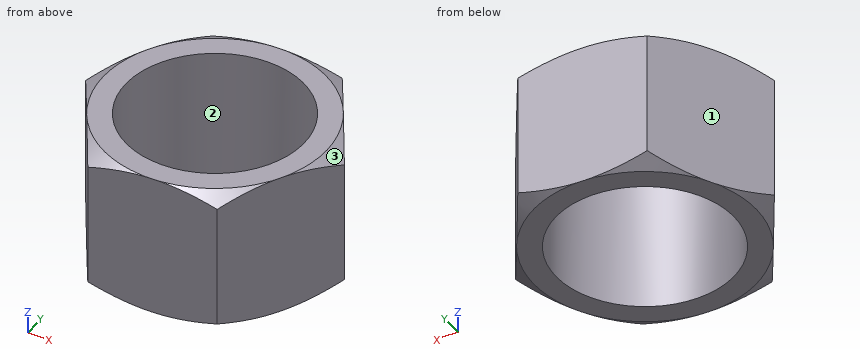
from build123d import *

# Parameters (mm, degrees)
SKETCH1_R           = 5
BOSS_EXTRUDE1_DEPTH = 8
SKETCH2_OUTSIDE_W   = 67.404
SKETCH2_OUTSIDE_H   = 65.714
SKETCH2_OUTSIDE_R   = 6.25
CUT_EXTRUDE1_DEPTH  = 13.512942035
CUT_EXTRUDE1_DRAFT  = -60
SKETCH3_OUTSIDE_W   = 67.404
SKETCH3_OUTSIDE_H   = 65.714
SKETCH3_OUTSIDE_R   = 6.251224569
CUT_EXTRUDE2_DEPTH  = 13.512942035
CUT_EXTRUDE2_DRAFT  = -60


with BuildPart() as part:
    # Sketch1 → Boss-Extrude1 (new body)
    with BuildSketch(Plane.XY):
        Polygon((3.396178054, 6.367833851), (-3.816616855, 6.125093396), (-7.212794909, -0.242740455), (-3.396178054, -6.367833851), (3.816616855, -6.125093396), (7.212794909, 0.242740455), align=None)
        Circle(SKETCH1_R, mode=Mode.SUBTRACT)
    extrude(amount=BOSS_EXTRUDE1_DEPTH)


with BuildPart() as cut_extrude1_tool:
    # Sketch2 outside → Cut-Extrude1 (with draft: the straight prism first)
    with BuildSketch(Plane.XY.offset(8)):
        Rectangle(SKETCH2_OUTSIDE_W, SKETCH2_OUTSIDE_H)
        Circle(SKETCH2_OUTSIDE_R, mode=Mode.SUBTRACT)
    extrude(amount=-CUT_EXTRUDE1_DEPTH)
    # Cut-Extrude1: the draft: its side faces are tilted about the plane it starts from
    cut_extrude1_sides = [cut_extrude1_tool.faces().sort_by_distance(p)[0] for p in [
        (0, -32.857, 1.243528983),
        (33.702, 0, 1.243528983),
        (0, 32.857, 1.243528983),
        (-33.702, 0, 1.243528983),
        (-6.25, 0, 1.243528983),
    ]]
    draft(cut_extrude1_sides, Plane.XY.offset(8), CUT_EXTRUDE1_DRAFT)


with BuildPart() as part_1:
    add(part.part)

    # Cut-Extrude1: cut by cut_extrude1_tool
    add(cut_extrude1_tool.part, mode=Mode.SUBTRACT)


with BuildPart() as cut_extrude2_tool:
    # Sketch3 outside → Cut-Extrude2 (with draft: the straight prism first)
    with BuildSketch(Plane(origin=(0, 0, 0), x_dir=(-1, 0, 0), z_dir=(0, 0, -1))):
        Rectangle(SKETCH3_OUTSIDE_W, SKETCH3_OUTSIDE_H)
        Circle(SKETCH3_OUTSIDE_R, mode=Mode.SUBTRACT)
    extrude(amount=-CUT_EXTRUDE2_DEPTH)
    # Cut-Extrude2: the draft: its side faces are tilted about the plane it starts from
    cut_extrude2_sides = [cut_extrude2_tool.faces().sort_by_distance(p)[0] for p in [
        (0, -32.857, 6.756471017),
        (-33.702, 0, 6.756471017),
        (0, 32.857, 6.756471017),
        (33.702, 0, 6.756471017),
        (6.251224569, 0, 6.756471017),
    ]]
    draft(cut_extrude2_sides, Plane(origin=(0, 0, 0), x_dir=(-1, 0, 0), z_dir=(0, 0, -1)), CUT_EXTRUDE2_DRAFT)


with BuildPart() as part_2:
    add(part_1.part)

    # Cut-Extrude2: cut by cut_extrude2_tool
    add(cut_extrude2_tool.part, mode=Mode.SUBTRACT)


solid = part_2.part
Here's how the part is built. I have some questions about the finished solid (model axes, mm). Face numbers are marked on the shaded views. Coordinates: 2 decimals unless noted, no trailing zeros. Write each loop counter-clockwise with the first axis right and the second up, starting at its lowest first coordinate (ties: lowest second). Pieces come first, ordered by that corner, then holes.
1) I'm going to push flat-ended pins straight in: pin 1 (1.5 mm diameter, centred on y = -3, z = 1.5, fed in from -X); pin 2 (2 mm diameter, centred on x = 2.5, z = 4.5, fed in from +Y); pin 3 (3 mm diameter, centred on x = -2.5, z = 4, fed in from +Y). Where does each tip first touch, or does it pass through?
Filled in:
pin 1: stops at x = -5.96
pin 2: stops at y = 6.37
pin 3: stops at y = 6.22
2) Thinking about a two-plate mould opening in X: for the marked faces 1, 2 and 3, which applies, +X half, -X half, draft (parallel to the pull), parting line (faces both ways), or undercut?
Filled in:
face 1: -X half
face 2: undercut
face 3: +X half
3) If I drill on line 1 (Y direction, x = 0, z = 3.5); line 2 (X direction, y = 3.25, z = 5); line 3 (X direction, y = -3.25, z = 7.5), over which ranges is the centre line in solid material (lowest first)?
Filled in:
line 1: y = -6.25 to -5, 5 to 6.25
line 2: x = -5.35 to -3.8, 3.8 to 5.34
line 3: x = -5.34 to -3.8, 3.8 to 5.35
4) If we section it at B-B (y = 0): List the corners of the cut face in (x, z) for me, plus the area to 3 significant figures.
Filled in:
outline: (-7.08, 0.48) - (-6.25, 0) - (-5, 0) - (-5, 8) - (-6.25, 8) - (-7.08, 7.52) - close; (5, 0) - (6.25, 0) - (7.08, 0.48) - (7.08, 7.52) - (6.25, 8) - (5, 8) - close
area: 32.5 mm2
5) If we section it at A-A (z = 3): List the corners of the cut face in (x, y) for me, plus the area to 3 significant figures.
Filled in:
outline: (-7.21, -0.24) - (-3.4, -6.37) - (3.82, -6.13) - (7.21, 0.24) - (3.4, 6.37) - (-3.82, 6.13) - close; hole circle Ø10 at (0, 0)
area: 56.8 mm2
